from build123d import *

# Parameters (mm, degrees)
F0_R     = 1.397
F1_DEPTH = 3.429
F2_W     = 20.2819
F2_H     = 4.191
F3_DEPTH = 16.8275
F4_R     = 1.3335
F5_DEPTH = 12.7


with BuildPart() as f1:
    # F0 (on Front) → F1 (new body)
    with BuildSketch(Plane.XZ):
        Polygon((0, 10.16), (0, 0), (20.2819, 0), (20.2819, 10.16), (10.14095, 10.16), align=None)
        with Locations((2.3495, 3.5179)):
            Circle(F0_R, mode=Mode.SUBTRACT)
        with BuildLine():
            ThreePointArc((18.9865, 3.5179), (17.5895, 2.1209), (16.1925, 3.5179))
            ThreePointArc((16.1925, 3.5179), (17.5895, 4.9149), (18.9865, 3.5179))
        make_face(mode=Mode.SUBTRACT)
    extrude(amount=F1_DEPTH)

    # F2 (on face) → F3 (join)
    with BuildSketch(Plane.XZ.offset(3.429)):
        with Locations((10.14095, 8.0645)):
            Rectangle(F2_W, F2_H)
    extrude(amount=F3_DEPTH)

    # F4 (on face) → F5 (cut, symmetric)
    with BuildSketch(Plane(origin=(0, 0, 5.969), x_dir=(1, 0, 0), z_dir=(0, 0, -1))):
        with Locations((15.10665, 4.064)):
            Circle(F4_R)
    extrude(amount=F5_DEPTH, both=True, mode=Mode.SUBTRACT)


solid = f1.part
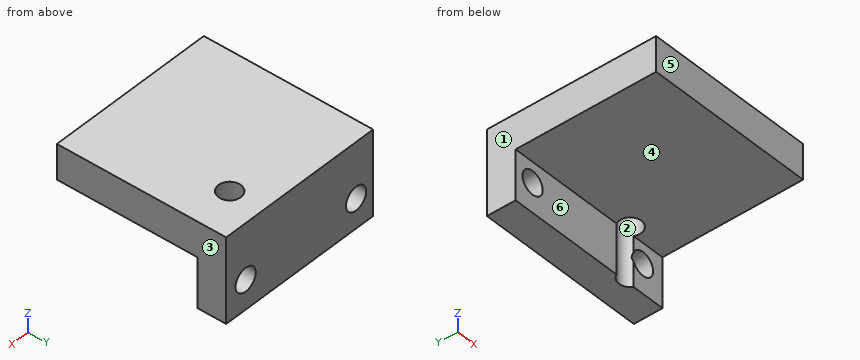
Verification items for the finished model (mm, model axes). Face numbers are marked on the shaded views. A direction names the side the tool comes from. Coordinates: 2 decimals unless noted, no trailing zeros. Order: outer loops, then holes, each group sorted by start corner. A loop starts at its lowest first (then second) coordinate and runs counter-clockwise, first axis right, second up. Notation, with made-up numbers: M -22,-17 L 22,-17 A22 cw 22,13 Z; hole C 40.5,46 d5. An arc over 180 degrees is marked long. One line per item, written item: value. Start each with the question number.
Item 1: Mould release check, pull along X, two halves, no side actions. Record for the marked faces 1, 2, 3 and 4: released by +X, released by -X, zero draft, split by the parting line, or undercut.
Item 2: Scan lines: probe 1 along X at (y, z) = (-2.5, 2.25); probe 2 along Z at (x, y) = (18, -19); probe 3 along Y at (x, z) = (9, 2.25). Record each from-to range of solid material in increasing order.
Item 3: Gauge pin test, flat ends, axial feed: pin 1 (2 mm diameter, centred on x = 15.11, y = -4.06, fed in from +Z); pin 2 (5 mm diameter, centred on x = 6, y = -13, fed in from -Z); pin 3 (4.5 mm diameter, centred on x = 18.5, z = 2.5, fed in from -Y). Record the tip position at first contact, or that the pin passes through.
Item 4: Sectioned sample at B-B (y = -1.75). Enter the section's corners in (x, z).
Item 5: Access from +Z, -Z, +X, -X, +Y, -Y to the whole of each face (thin tool, end or side, straight path). Record for the marked faces 5 and 6.
Item 6: Sectioned sample at D-D (y = -8). Enter the section's corners in (x, z), then the cut area to 3 significant figures.
Item 7: Sectioned sample at C-C (z = 5.5). Enter the section's corners in (x, y).
Item 8: Sectioned sample at A-A (x = 18.25). Enter the section's corners in (y, z).
Conclusion:
1. face 1: released by -X
1. face 2: undercut
1. face 3: released by +X
1. face 4: zero draft
2. probe 1: x = 0 to 1.76, 2.94 to 17, 18.18 to 20.28
2. probe 2: z = 5.97 to 10.16
2. probe 3: y = -3.43 to 0
3. pin 1: passes through
3. pin 2: stops at z = 5.97
3. pin 3: stops at y = -3.43
4. outline: M 0,0 L 20.28,0 L 20.28,10.16 L 0,10.16 Z; hole C 2.35,3.52 d2.79; hole C 17.59,3.52 d2.79
5. face 5: +Z, -Z, +X, -X, -Y
5. face 6: -Z, +X, -X, -Y
6. outline: M 0,5.97 L 20.28,5.97 L 20.28,10.16 L 0,10.16 Z
6. area: 85.0 mm^2
7. outline: M 0,-3.43 L 13.93,-3.43 A1.33 cw 16.28,-3.43 L 20.28,-3.43 L 20.28,0 L 0,0 Z
8. outline: M -20.26,5.97 L -3.43,5.97 L -3.43,4.75 L 0,4.75 L 0,10.16 L -20.26,10.16 Z; M -3.43,0 L 0,0 L 0,2.29 L -3.43,2.29 Z
